Work out the finished part from the listing and answer in its coordinate system (mm). Face numbers are marked on the shaded views. Coordinates: 2 decimals unless noted, no trailing zeros. Order: outer loops, then holes, each group sorted by start corner. A loop starts at its lowest first (then second) coordinate and runs counter-clockwise, first axis right, second up. Notation, with made-up numbers: M -27.5,39.25 L 0.5,39.25 A35 ccw 0.5,74.25 Z; hole C 67.5,42 d1. An arc over 180 degrees is marked long. Answer in a Markdown table with one row per item. Add a question column.
Item 1: Consider line 1 (Y direction, x = 0, z = -1.25); line 2 (Z direction, x = 4, y = -3.25); line 3 (X direction, y = -2.75, z = -3). Determine where each line is inside the solid, lowest interval first. Write a range as from..to.
Item 2: Flat-ended cylindrical pins translate along their axes: pin 1 Ø1 at (y, z) = (-2, -7.5) entering from +X; pin 2 Ø2 at (x, y) = (-1, 1.5) entering from +Z; pin 3 Ø1 at (y, z) = (1, -4) entering from -X. Find the tip coordinate at first contact, or state that the pin passes through.
Item 3: The part is cut by section D-D (z = -1.5). Write down the section's boundary in (x, y), then the cut area to 3 significant figures.
Item 4: The part is cut by section C-C (z = -7). Write down the section's boundary in (x, y).
Item 5: The part is cut by section A-A (y = 0). Write down the section's boundary in (x, z), then the cut area to 3 significant figures.
Item 6: The mould has two halves that part along X. Classify the marked faces 1, 2 and 3: released by +X, released by -X, zero draft, split by the parting line, or undercut.
from build123d import *

# Parameters (mm, degrees)
SKETCH1_R           = 5.5
BOSS_EXTRUDE1_DEPTH = 2
SKETCH2_R           = 4.25
BOSS_EXTRUDE2_DEPTH = 7
SKETCH5_R           = 3.5
CUT_EXTRUDE3_DEPTH  = 8


with BuildPart() as part:
    # Sketch1 → Boss-Extrude1 (new body)
    with BuildSketch(Plane.XY):
        Circle(SKETCH1_R)
    extrude(amount=-BOSS_EXTRUDE1_DEPTH)

    # Sketch2 → Boss-Extrude2 (add)
    with BuildSketch(Plane(origin=(0, 0, -2), x_dir=(-1, 0, 0), z_dir=(0, 0, -1))):
        Circle(SKETCH2_R)
    extrude(amount=BOSS_EXTRUDE2_DEPTH)

    # Sketch5 → Cut-Extrude3 (cut)
    with BuildSketch(Plane.XY):
        Circle(SKETCH5_R)
    extrude(amount=-CUT_EXTRUDE3_DEPTH, mode=Mode.SUBTRACT)


solid = part.part
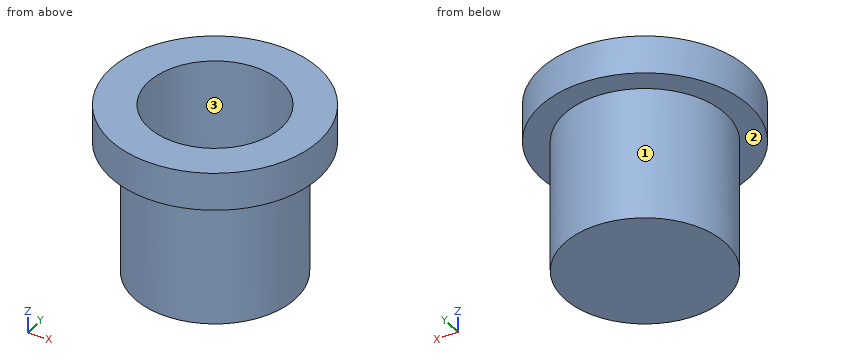
Reply:
| question | item | result |
|---|---|---|
| 1 | line 1 | y = -5.5..-3.5, 3.5..5.5 |
| 1 | line 2 | z = -2..0 |
| 1 | line 3 | x = -3.24..-2.17, 2.17..3.24 |
| 2 | pin 1 | stops at x = 3.98 |
| 2 | pin 2 | stops at z = -8 |
| 2 | pin 3 | stops at x = -4.22 |
| 3 | outline | C 0,0 d11; hole C 0,0 d7 |
| 3 | area | 56.5 mm2 |
| 4 | outline | C 0,0 d8.5; hole C 0,0 d7 |
| 5 | outline | M -5.5,-2 L -4.25,-2 L -4.25,-9 L 4.25,-9 L 4.25,-2 L 5.5,-2 L 5.5,0 L 3.5,0 L 3.5,-8 L -3.5,-8 L -3.5,0 L -5.5,0 Z |
| 5 | area | 25.5 mm2 |
| 6 | face 1 | split by the parting line |
| 6 | face 2 | zero draft |
| 6 | face 3 | undercut |
